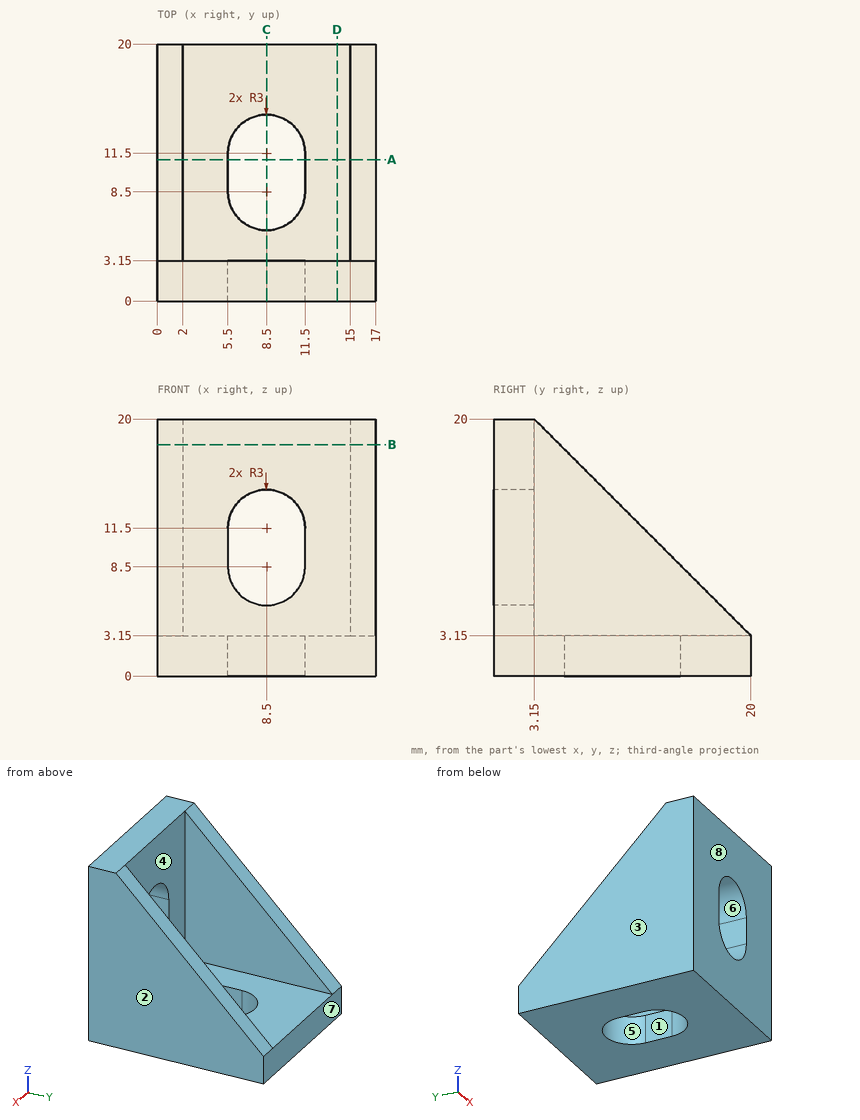
Answer from the drawing. Dimensions are ordinates in mm from the lowest x, y and z of the part. A direction names the side the tool comes from. Give positions to 0.01 mm unless a question says otherwise; leave off trailing zeros. Loops run counter-clockwise (first coordinate to the right, second up) from the corner with the lowest first, then second, coordinate; pieces in that order, holes last. Notation, with made-up numbers: (-36, 3.5) -> (-22, 3.5) arc R16 cw to (-22, 30.5) -> close; hole circle Ø9 at (63, 67). An arc over 180 degrees is marked (long way). Answer as CSV lines item,"result".
Item 1: Find section A-A on y = 11. Give the vertices of the cut face in (x, z).
Returned:
outline,"(0, 0) -> (5.5, 0) -> (5.5, 3.15) -> (2, 3.15) -> (2, 12.15) -> (0, 12.15) -> close; (11.5, 0) -> (17, 0) -> (17, 12.15) -> (15, 12.15) -> (15, 3.15) -> (11.5, 3.15) -> close"
Item 2: Consider line 1 (X direction, y = 10.75, z = 6.5); line 2 (Y direction, x = 12.5, z = 8.25). Determine where each line is inside the solid, lowest interval first. Write a range as [from, to].
Returned:
line 1,"x = [0, 2], [15, 17]"
line 2,"y = [0, 3.15]"
Item 3: Determine the mould class of the marked faces 1, 2 and 3 for opening direction X: +X half, -X half, draft (parallel to the pull), parting line (faces both ways), or undercut.
Returned:
face 1,"undercut"
face 2,"+X half"
face 3,"-X half"
Item 4: Find section D-D on x = 14. Give the vertices of the cut face in (y, z), plus the area to 3 significant figures.
Returned:
outline,"(0, 0) -> (20, 0) -> (20, 3.15) -> (3.15, 3.15) -> (3.15, 20) -> (0, 20) -> close"
area,"116 mm²"
Item 5: Find section B-B on z = 18. Give the vertices of the cut face in (x, y), plus the area to 4 significant figures.
Returned:
outline,"(0, 0) -> (17, 0) -> (17, 5.15) -> (15, 5.15) -> (15, 3.15) -> (2, 3.15) -> (2, 5.15) -> (0, 5.15) -> close"
area,"61.55 mm²"
Item 6: Find section C-C on x = 8.5. Give the vertices of the cut face in (y, z).
Returned:
outline,"(0, 0) -> (5.5, 0) -> (5.5, 3.15) -> (3.15, 3.15) -> (3.15, 5.5) -> (0, 5.5) -> close; (0, 14.5) -> (3.15, 14.5) -> (3.15, 20) -> (0, 20) -> close; (14.5, 0) -> (20, 0) -> (20, 3.15) -> (14.5, 3.15) -> close"
Item 7: Each of these flat-tipped pins is pushed along its axis until it touches: pin 1 (6 mm diameter, centred on y = 16, z = 15, fed in from +X); pin 2 (6.5 mm diameter, centred on x = 10.5, y = 14, fed in from +Z). Where does it stop, or does it pass through?
Returned:
pin 1,"passes through"
pin 2,"stops at z = 3.15"
Item 8: For the marked faces 4, 5, 6, 7 and 8, determine the directions among +Z, -Z, +X, -X, +Y, -Y from which every point of the face is accessible in a straight line to the end or side of a thin tool.
Returned:
face 4,"+Z, +Y"
face 5,"+Z, -Z"
face 6,"+Y, -Y"
face 7,"+Z, -Z, +X, -X, +Y"
face 8,"+Z, -Z, +X, -X, -Y"
